Geometry: final body of the model. Coordinates: model frame, mm. A direction names the side the tool comes from. Round coordinates to 2 decimals unless told otherwise and drop trailing zeros. Write each loop counter-clockwise with the first axis right and the second up, starting at its lowest first coordinate (ties: lowest second). Pieces come first, ordered by that corner, then holes. Notation, with made-up numbers: M 31,-17.5 L 63,-17.5 A18 cw 63,14.5 Z; hole C -33,30 d10. An arc over 180 degrees is marked long. Put each result on its own line as item: value. Start each with the question number.
```python
from build123d import *

# Parameters (mm, degrees)
CROQUIS1_W              = 66.01
CROQUIS1_H              = 21
SALIENTE_EXTRUIR1_DEPTH = 1
CROQUIS2_W              = 66.01
CROQUIS2_H              = 21
CROQUIS2_W_2            = 64.01
CROQUIS2_H_2            = 19
SALIENTE_EXTRUIR2_DEPTH = 1
SALIENTE_EXTRUIR3_REACH = 4
CROQUIS5_R              = 0.6
CORTAR_EXTRUIR1_DEPTH   = 3
CROQUIS6_R              = 1.1
CORTAR_EXTRUIR2_DEPTH   = 1
REDONDEO1_R             = 1


with BuildPart() as part:
    # Croquis1 → Saliente-Extruir1 (new body)
    with BuildSketch(Plane(origin=(0, 0, 0), x_dir=(1, 0, 0), z_dir=(0, 1, 0))):
        with Locations((33.005, 10.5)):
            Rectangle(CROQUIS1_W, CROQUIS1_H)
    extrude(amount=SALIENTE_EXTRUIR1_DEPTH)

    # Croquis2 → Saliente-Extruir2 (add)
    with BuildSketch(Plane(origin=(0, 1, 0), x_dir=(1, 0, 0), z_dir=(0, 1, 0))):
        with Locations((33.005, 10.5)):
            Rectangle(CROQUIS2_W, CROQUIS2_H)
        with Locations((33.005, 10.5)):
            Rectangle(CROQUIS2_W_2, CROQUIS2_H_2, mode=Mode.SUBTRACT)
    extrude(amount=SALIENTE_EXTRUIR2_DEPTH)

    # Croquis4 → Saliente-Extruir3 (add, up to next)
    with BuildSketch(Plane(origin=(0, 2, 0), x_dir=(1, 0, 0), z_dir=(0, 1, 0)), mode=Mode.PRIVATE) as saliente_extruir3_sk1:
        with BuildLine():
            Line((1, 20), (1, 17.85))
            ThreePointArc((1, 17.85), (2.52027958, 18.47972042), (3.15, 20))
            Line((3.15, 20), (1, 20))
        make_face()
    saliente_extruir3_tool1 = extrude(saliente_extruir3_sk1.sketch, amount=-SALIENTE_EXTRUIR3_REACH, mode=Mode.PRIVATE) - part.part
    add(saliente_extruir3_tool1.solids().sort_by_distance((1.912488, 2, -19.087512))[0])
    # Croquis4 → Saliente-Extruir3 (add, up to next)
    with BuildSketch(Plane(origin=(0, 2, 0), x_dir=(1, 0, 0), z_dir=(0, 1, 0)), mode=Mode.PRIVATE) as saliente_extruir3_sk2:
        with BuildLine():
            Line((1, 1), (1, 3.15))
            ThreePointArc((1, 3.15), (2.52027958, 2.52027958), (3.15, 1))
            Line((3.15, 1), (1, 1))
        make_face()
    saliente_extruir3_tool2 = extrude(saliente_extruir3_sk2.sketch, amount=-SALIENTE_EXTRUIR3_REACH, mode=Mode.PRIVATE) - part.part
    add(saliente_extruir3_tool2.solids().sort_by_distance((1.912488, 2, -1.912488))[0])
    # Croquis4 → Saliente-Extruir3 (add, up to next)
    with BuildSketch(Plane(origin=(0, 2, 0), x_dir=(1, 0, 0), z_dir=(0, 1, 0)), mode=Mode.PRIVATE) as saliente_extruir3_sk3:
        with BuildLine():
            Line((65.01, 20), (62.86, 20))
            ThreePointArc((62.86, 20), (63.48972042, 18.47972042), (65.01, 17.85))
            Line((65.01, 17.85), (65.01, 20))
        make_face()
    saliente_extruir3_tool3 = extrude(saliente_extruir3_sk3.sketch, amount=-SALIENTE_EXTRUIR3_REACH, mode=Mode.PRIVATE) - part.part
    add(saliente_extruir3_tool3.solids().sort_by_distance((64.097512, 2, -19.087512))[0])
    # Croquis4 → Saliente-Extruir3 (add, up to next)
    with BuildSketch(Plane(origin=(0, 2, 0), x_dir=(1, 0, 0), z_dir=(0, 1, 0)), mode=Mode.PRIVATE) as saliente_extruir3_sk4:
        with BuildLine():
            Line((65.01, 1), (62.86, 1))
            ThreePointArc((62.86, 1), (63.48972042, 2.52027958), (65.01, 3.15))
            Line((65.01, 3.15), (65.01, 1))
        make_face()
    saliente_extruir3_tool4 = extrude(saliente_extruir3_sk4.sketch, amount=-SALIENTE_EXTRUIR3_REACH, mode=Mode.PRIVATE) - part.part
    add(saliente_extruir3_tool4.solids().sort_by_distance((64.097512, 2, -1.912488))[0])

    # Croquis5 → Cortar-Extruir1 (cut, through all)
    with BuildSketch(Plane(origin=(0, 2, 0), x_dir=(1, 0, 0), z_dir=(0, 1, 0))):
        with Locations((1.76013979, 19.23986021)):
            Circle(CROQUIS5_R)
        with Locations((1.76013979, 1.76013979)):
            Circle(CROQUIS5_R)
        with Locations((64.24986021, 19.23986021)):
            Circle(CROQUIS5_R)
        with Locations((64.24986021, 1.76013979)):
            Circle(CROQUIS5_R)
    extrude(amount=-CORTAR_EXTRUIR1_DEPTH, mode=Mode.SUBTRACT)

    # Croquis6 → Cortar-Extruir2 (cut)
    with BuildSketch(Plane(origin=(0, 0, 0), x_dir=(-1, 0, 0), z_dir=(0, -1, 0))):
        with Locations((-64.24986021, 1.76013979)):
            Circle(CROQUIS6_R)
        with Locations((-64.24986021, 19.23986021)):
            Circle(CROQUIS6_R)
        with Locations((-1.76013979, 19.23986021)):
            Circle(CROQUIS6_R)
        with Locations((-1.76013979, 1.76013979)):
            Circle(CROQUIS6_R)
    extrude(amount=-CORTAR_EXTRUIR2_DEPTH, mode=Mode.SUBTRACT)

    # Redondeo1
    redondeo1_edges = [part.edges().sort_by_distance(p)[0] for p in [
        (0, 1, -21),
        (66.01, 1, -21),
        (66.01, 1, 0),
        (0, 1, 0),
    ]]
    fillet(redondeo1_edges, radius=REDONDEO1_R)


solid = part.part
```
1) First-contact query: pin 1 (2 mm diameter, centred on x = 1.76, z = -19.24, fed in from -Y); pin 2 (4 mm diameter, centred on x = 11, z = -12.5, fed in from +Y); pin 3 (0.7 mm diameter, centred on x = 64.25, z = -19.24, fed in from +Y) (3 decimals). Flat tips, straight axial feed; report the tip coordinate or a pass-through.
2) Ray query, probe 1 along X at (y, z) = (1.4, -13.25); probe 2 along Z at (x, y) = (47, 1.05); probe 3 along Y at (x, z) = (18.5, -12.5). Return the intervals inside material, ascending.
3) Access query for faces 4 (the face through (64, 1, -1)), 5 (the face through (1.682, 1.507, -19.835)), 6 (the face through (33, 1, -11)). Directions: +Z, -Z, +X, -X, +Y, -Y. A direction counts if a zero-diameter tool reaches every point of the face in a straight line with its end or side. Return the directions, or none.
4) Section A-A, the plane z = -14. Output: boundary loops of the cut face in (x, y).
5) Draft query along Z for faces 1 (the face through (33, 0, -11)), 2 (the face through (33, 1, -21)), 3 (the face through (63.77, 1.51, -1.4)). Return one class per face: +Z half, -Z half, draft (parallel to the pull), parting line (faces both ways), or undercut.
6) Section B-B, the plane x = 55. Output: boundary loops of the cut face in (y, z), and give its area (3 significant figures).
7) Section C-C, the plane y = 1.7. Output: boundary loops of the cut face in (x, z), and give its area (3 significant figures).
Solved:
1. pin 1: stops at y = 1
1. pin 2: stops at y = 1
1. pin 3: passes through
2. probe 1: x = 0 to 1, 65.01 to 66.01
2. probe 2: z = -21 to -20, -1 to 0
2. probe 3: y = 0 to 1
3. face 4: -Y
3. face 5: +Y, -Y
3. face 6: +Y
4. outline: M 0,0 L 66.01,0 L 66.01,2 L 65.01,2 L 65.01,1 L 1,1 L 1,2 L 0,2 Z
5. face 1: draft
5. face 2: -Z half
5. face 3: undercut
6. outline: M 0,-21 L 2,-21 L 2,-20 L 1,-20 L 1,-1 L 2,-1 L 2,0 L 0,0 Z
6. area: 23.0 mm2
7. outline: M 0,-20 A1 ccw 1,-21 L 65.01,-21 A1 ccw 66.01,-20 L 66.01,-1 A1 ccw 65.01,0 L 1,0 A1 ccw 0,-1 Z; hole M 1,-17.85 A2.15 cw 3.15,-20 L 62.86,-20 A2.15 cw 65.01,-17.85 L 65.01,-3.15 A2.15 cw 62.86,-1 L 3.15,-1 A2.15 cw 1,-3.15 Z; hole C 1.76,-19.24 d1.2; hole C 1.76,-1.76 d1.2; hole C 64.25,-19.24 d1.2; hole C 64.25,-1.76 d1.2
7. area: 179 mm2
